Build history of the part. All positions in model axes, mm. Face numbers are marked on the shaded views. A direction names the side the tool comes from. Give positions to 0.01 mm unless a question says otherwise; leave off trailing zeros. Loops run counter-clockwise (first coordinate to the right, second up) from the corner with the lowest first, then second, coordinate; pieces in that order, holes last. Notation, with made-up numbers: M 64,72.25 L 118,72.25 A23 cw 118,100.25 Z; hole C 73.25,-35 d8. An arc over 180 degrees is marked long. Answer in a Markdown table with one row per item. Add a question column.
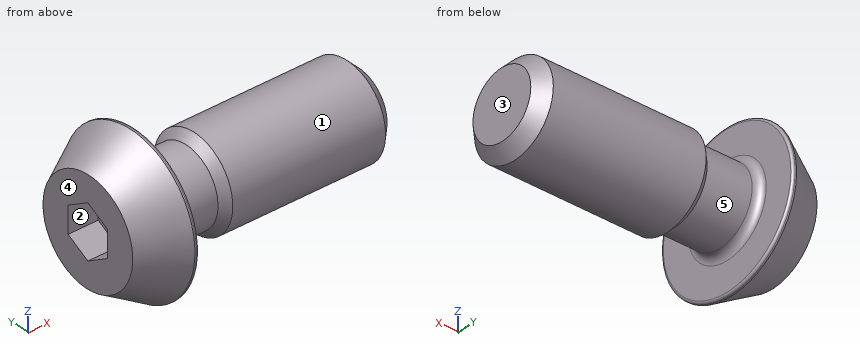
```python
from build123d import *

# Parameters (mm, degrees)
CUT_EXTRUDE_1_DEPTH = 4
FILLET_1_R          = 0.3
CHAMFER_1_SIZE      = 1.6
FILLET_2_R          = 1


with BuildPart() as part:
    # Эскиз1 → Повернуть1 (revolve)
    with BuildSketch(Plane.XY):
        Polygon((0, 0), (0, 6.824573519), (5.5, 10), (6, 10), (6, 4.95), (13, 4.95), (14.05, 6), (36, 6), (36, 0), align=None)
    revolve(axis=Axis((36, 0, 0), (-1, 0, 0)))

    # Эскиз2 → Вырез-Вытянуть1 (cut)
    with BuildSketch(Plane.ZY):
        Polygon((1.732050808, 3), (-1.732050808, 3), (-3.464101615, 0), (-1.732050808, -3), (1.732050808, -3), (3.464101615, 0), align=None)
    extrude(amount=-CUT_EXTRUDE_1_DEPTH, mode=Mode.SUBTRACT)

    # Скругление1
    fillet_1_edges = [part.edges().sort_by_distance(p)[0] for p in [
        (6, -10, 0),
    ]]
    fillet(fillet_1_edges, radius=FILLET_1_R)

    # Фаска1
    chamfer_1_edges = [part.edges().sort_by_distance(p)[0] for p in [
        (36, -6, 0),
    ]]
    chamfer(chamfer_1_edges, length=CHAMFER_1_SIZE)

    # Скругление2
    fillet_2_edges = [part.edges().sort_by_distance(p)[0] for p in [
        (6, -4.95, 0),
    ]]
    fillet(fillet_2_edges, radius=FILLET_2_R)


solid = part.part
```
(1) Wall check: line 1 (Y direction, x = 11, z = -2.25); line 2 (Z direction, x = 15, y = 0.25); line 3 (Z direction, x = 2.5, y = 0.25). Give the ranges that are in metal, low to high.
(2) Pin check, flat tips, straight feed: pin 1 (8 mm diameter, centred on x = 17, z = -4.5, fed in from +Y); pin 2 (12 mm diameter, centred on x = 13, y = 3.5, fed in from +Z); pin 3 (10 mm diameter, centred on x = 28.5, z = -5, fed in from -Y). Stop position of each tip, or through.
(3) Pull direction X, two halves, no side cores. Call the marked faces 3, 4 and 5: +X half, -X half, draft (parallel to the pull), parting line (faces both ways), or undercut.
(4) Tool access for the marked faces 1 and 2: list every direction of +Z, -Z, +X, -X, +Y, -Y with a clear straight run to the whole face (end or side of a thin tool).
(5) Slice it at C-C, the plane x = 8. Give the cut face in (y, z).
(6) Slice it at A-A, the plane z = 0. Give the cut face in (x, y), then the cut area to 3 significant figures.
(7) Slice it at B-B, the plane x = 15. Give the cut face in (y, z).
Solution:
| question | item | result |
|---|---|---|
| 1 | line 1 | -4.41 to 4.41 |
| 1 | line 2 | -5.99 to 5.99 |
| 1 | line 3 | -8.26 to -3.32, 3.32 to 8.26 |
| 2 | pin 1 | y = 5.98 |
| 2 | pin 2 | z = 6 |
| 2 | pin 3 | y = -6 |
| 3 | face 3 | +X half |
| 3 | face 4 | -X half |
| 3 | face 5 | undercut |
| 4 | face 1 | +X |
| 4 | face 2 | -X |
| 5 | outline | C 0,0 d9.9 |
| 6 | outline | M 0,-6.82 L 5.5,-10 L 5.7,-10 A0.3 ccw 6,-9.7 L 6,-5.95 A1 cw 7,-4.95 L 13,-4.95 L 14.05,-6 L 34.4,-6 L 36,-4.4 L 36,4.4 L 34.4,6 L 14.05,6 L 13,4.95 L 7,4.95 A1 cw 6,5.95 L 6,9.7 A0.3 ccw 5.7,10 L 5.5,10 L 0,6.82 L 0,3 L 4,3 L 4,-3 L 0,-3 Z |
| 6 | area | 421 mm^2 |
| 7 | outline | C 0,0 d12 |
